Autodesk Inventor part; units mm, degrees
ref_plane "YZ Plane" through (0, 0, 0) normal (1, 0, 0) x (0, 1, 0)
ref_plane "XZ Plane" through (0, 0, 0) normal (0, 1, 0) x (-1, 0, 0)
ref_plane "XY Plane" through (0, 0, 0) normal (0, 0, 1) x (1, 0, 0)
sketch "Sketch1" plane through (0, 0, 0) normal (0, 1, 0) x (-1, 0, 0)
  line L0 (0, 0) -> (0, 29.5)
  line L1 (25, 0) -> (25, 10)
  line L2 (25, 10) -> (23, 29.5)
  line L3 (23, 29.5) -> (21, 29.5)
  line L4 (22, 0) -> (25, 0)
  line L5 (0, 0) -> (22, 0) construction
  line L6 (21, 29.5) -> (0, 29.5) construction
  line L7 (21, 29.5) -> (21, 21.5)
  line L8 (21, 21.5) -> (22, 0)
  dimension "d0" = 50
  dimension "d1" = 42
  dimension "d2" = 29.5
  dimension "d3" = 10
  dimension "d4" = 8
  dimension "d11" = 3
  dimension "d12" = 2
revolve "Revolution1" add sketch "Sketch1" angle 360 about axis through (0, 0, 0) along (0, 0, 1)
chamfer "Chamfer1" distance 0.5 angle 45 4 edges at (25, 0, 0) (22, 0, 0) (23, 0, 29.5) (21, 0, 29.5)
properties part number "TakumarSpacer" material "ABS Plastic"
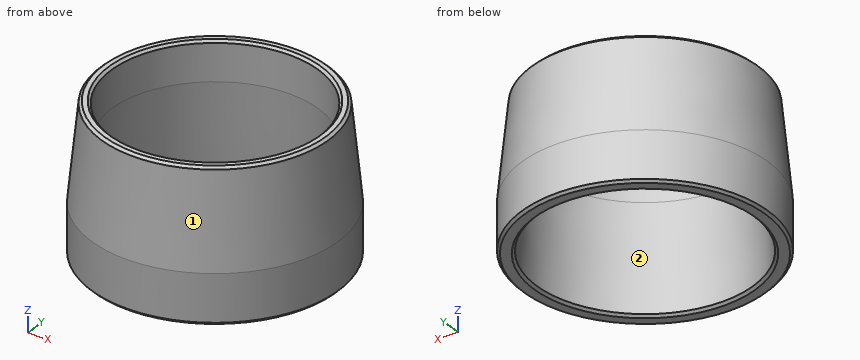
For this review, take the finished solid that the model builds, in its own axes (mm). Face numbers are marked on the shaded views. Round coordinates to 2 decimals unless told otherwise and drop trailing zeros. Write each loop counter-clockwise with the first axis right and the second up, starting at its lowest first coordinate (ties: lowest second). Pieces come first, ordered by that corner, then holes. Notation, with made-up numbers: (75, 44.25) - (86, 44.25) arc R24 ccw to (86, 58.25) - close; hole circle Ø3 at (82, 25). An arc over 180 degrees is marked (long way). Write item = value, one per line. Start each with the question number.
1. Draft analysis for pull direction X (two halves, no side actions). For the marked faces 1 and 2, state which applies: released by +X, released by -X, zero draft, split by the parting line, or undercut.
2. Consider section D-D on z = 16.5. State the section outline as (x, y) points, plus the area to 3 significant figures.
3. Wall thickness on L1, parallel to X at y = 0, z = 25.5; L2, parallel to X at y = -16, z = 20.5; L3, parallel to Y at x = 19, z = 9.5: over which ranges is each line inside the solid? List them lowest first.
4. For pin 1 Ø8 at (y, z) = (11, 10.5) entering from -X; pin 2 Ø10 at (x, z) = (-2, 24.5) entering from -Y; pin 3 Ø1 at (y, z) = (-10, 17) entering from +X, all flat-tipped, find the tip position at first contact; note any pin that passes through.
5. Consider section C-C on z = 4. State the section outline as (x, y) points.
6. Consider section A-A on y = 0. State the section outline as (x, z) points.
Evaluation:
q1.face_1 = split by the parting line
q1.face_2 = undercut
q2.outline = circle Ø48.67 at (0, 0); hole circle Ø42.47 at (0, 0)
q2.area = 444 mm2
q3.L1 = -23.41 to -21, 21 to 23.41
q3.L2 = -17.79 to -13.67, 13.67 to 17.79
q3.L3 = -16.25 to -10.19, 10.19 to 16.25
q4.pin_1 = -23.99
q4.pin_2 = -24
q4.pin_3 = 22.35
q5.outline = circle Ø50 at (0, 0); hole circle Ø43.63 at (0, 0)
q6.outline = (-25, 0.5) - (-24.5, 0) - (-22.5, 0) - (-21.98, 0.5) - (-21, 21.5) - (-21, 29) - (-21.5, 29.5) - (-22.5, 29.5) - (-23.05, 29) - (-25, 10) - close; (21, 21.5) - (21.98, 0.5) - (22.5, 0) - (24.5, 0) - (25, 0.5) - (25, 10) - (23.05, 29) - (22.5, 29.5) - (21.5, 29.5) - (21, 29) - close
